from build123d import *

# Parameters (mm, degrees)
BOSS_EXTRUDE1_DEPTH = 18
SKETCH2_W           = 42
SKETCH2_H           = 13
CUT_EXTRUDE1_DEPTH  = 42.832217781


with BuildPart() as part:
    # Sketch1 → Boss-Extrude1 (new body)
    with BuildSketch(Plane(origin=(0, 0, 0), x_dir=(1, 0, 0), z_dir=(0, 1, 0))):
        Polygon((-10.366666667, 24.383333333), (32.633333333, 24.383333333), (32.633333333, -0.616666667), (21.633333333, -0.616666667), (21.633333333, 18.383333333), (-10.366666667, 18.383333333), align=None)
    extrude(amount=BOSS_EXTRUDE1_DEPTH)

    # Sketch2 → Cut-Extrude1 (cut, through all)
    with BuildSketch(Plane.XY.offset(-18.383333333)):
        with Locations((-10.366666667, 9)):
            Rectangle(SKETCH2_W, SKETCH2_H)
    extrude(amount=-CUT_EXTRUDE1_DEPTH, mode=Mode.SUBTRACT)


solid = part.part
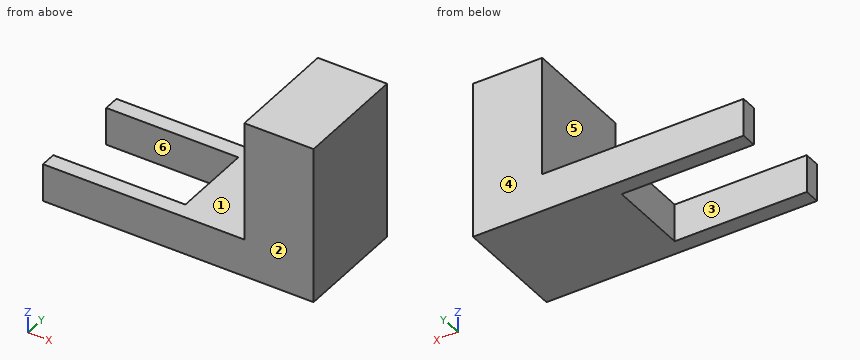
Geometry check sheet. Reference: the model listing, model coordinates, mm. Face numbers are marked on the shaded views. A direction names the side the tool comes from. Round coordinates to 2 decimals unless told otherwise and drop trailing zeros. Order: outer loops, then holes, each group sorted by start corner. A loop starts at its lowest first (then second) coordinate and runs counter-clockwise, first axis right, second up. Notation, with made-up numbers: M 21.5,77.5 L 44.5,77.5 A27 cw 44.5,94.5 Z; hole C 10.25,2.25 d8. An arc over 180 degrees is marked long. Answer in a Markdown table with one row per item. Add a question column.
Item 1: Set-up check for the marked faces 1, 2 and 3: record each of +Z, -Z, +X, -X, +Y, -Y from which the full face is reachable in a straight line by a thin tool's end or side.
Item 2: Sectioned sample at C-C, the plane y = 1. Enter the section's corners in (x, z).
Item 3: Depth check by flat-ended pin: pin 1 Ø3 at (y, z) = (10.5, -22) entering from -X; pin 2 Ø12 at (x, z) = (11.5, -8) entering from +Y; pin 3 Ø3 at (y, z) = (4.5, -15) entering from -X. Enter the tip coordinate at first touch or a pass-through.
Item 4: Sectioned sample at A-A, the plane x = 4. Enter the section's corners in (y, z), plus the area to 3 significant figures.
Item 5: Sectioned sample at B-B, the plane z = -20. Enter the section's corners in (x, y), plus the area to 3 significant figures.
Item 6: Draft check along Y on the marked faces 4, 5 and 6. Enter one of: released by +Y, released by -Y, zero draft, split by the parting line, or undercut.
Item 7: Sectioned sample at D-D, the plane x = 21. Enter the section's corners in (y, z), plus the area to 3 significant figures.
Item 8: Material ranges on L1, parallel to Y at x = -7.5, z = -21.5; L2, parallel to X at y = 15.5, z = -1.5; L3, parallel to X at y = 14, z = -22, recorded low to high. Write a range as [from, to].
Filled in:
| question | item | result |
|---|---|---|
| 1 | face 1 | +Z, -X, +Y, -Y |
| 1 | face 2 | +Z, -Z, +X, -X, -Y |
| 1 | face 3 | +Z, -Z, -X |
| 2 | outline | M -10.37,-24.38 L 32.63,-24.38 L 32.63,0.62 L 21.63,0.62 L 21.63,-18.38 L -10.37,-18.38 Z |
| 3 | pin 1 | stops at x = 10.63 |
| 3 | pin 2 | passes through |
| 3 | pin 3 | stops at x = 21.63 |
| 4 | outline | M 0,-24.38 L 2.5,-24.38 L 2.5,-18.38 L 0,-18.38 Z; M 15.5,-24.38 L 18,-24.38 L 18,-18.38 L 15.5,-18.38 Z |
| 4 | area | 30.0 mm² |
| 5 | outline | M -10.37,0 L 32.63,0 L 32.63,18 L -10.37,18 L -10.37,15.5 L 10.63,15.5 L 10.63,2.5 L -10.37,2.5 Z |
| 5 | area | 501 mm² |
| 6 | face 4 | released by +Y |
| 6 | face 5 | zero draft |
| 6 | face 6 | undercut |
| 7 | outline | M 0,-24.38 L 18,-24.38 L 18,-18.38 L 0,-18.38 Z |
| 7 | area | 108 mm² |
| 8 | L1 | y = [0, 2.5], [15.5, 18] |
| 8 | L2 | x = [21.63, 32.63] |
| 8 | L3 | x = [10.63, 32.63] |
